from build123d import *

# Parameters (mm, degrees)
F1_DEPTH = 25.4
F4_DEPTH = 15.875


with BuildPart() as f1:
    # F0 (on Front) → F1 (new body)
    with BuildSketch(Plane.XZ):
        with BuildLine():
            Line((1860.5442472816, 17.4135072052), (-120.6557527184, 17.4135072052))
            Line((-120.6557527184, 17.4135072052), (-120.6557527184, -58.7864927948))
            ThreePointArc((-120.6557527184, -58.7864927948), (869.9442472816, -7.9864927948), (1860.5442472816, -58.7864927948))
            Line((1860.5442472816, -58.7864927948), (1860.5442472816, 17.4135072052))
        make_face()
    extrude(amount=F1_DEPTH)


with BuildPart() as f4:
    # F3 (on Front) → F4 (new body)
    with BuildSketch(Plane.XZ):
        with BuildLine():
            Line((1910.8698048711, -377.0609709263), (-70.3301951289, -377.0609709263))
            Line((-70.3301951289, -377.0609709263), (-70.3301951289, -478.6609709263))
            ThreePointArc((-70.3301951289, -478.6609709262), (920.2698048711, -427.8609709262), (1910.8698048711, -478.6609709262))
            Line((1910.8698048711, -478.6609709263), (1910.8698048711, -377.0609709263))
        make_face()
    extrude(amount=F4_DEPTH)


solid = f4.part
Source: CAD feature listing. Evaluate the final solid. Frame: model axes, mm. Coordinates: 2 decimals unless noted, no trailing zeros. Write each loop counter-clockwise with the first axis right and the second up, starting at its lowest first coordinate (ties: lowest second). Pieces come first, ordered by that corner, then holes. Notation, with made-up numbers: M -25.75,87.5 L -19.75,87.5 A19 ccw -19.75,91.5 Z; hole C 62,-10 d8. An arc over 180 degrees is marked long. Use a Markdown table: item, result.
1) Ray query, L1, parallel to Z at x = 938, y = -7.25; L2, parallel to Z at x = 48, y = -2.25. Return the intervals inside material, ascending.
Conclusion:
| item | result |
|---|---|
| L1 | z = -427.88 to -377.06 |
| L2 | z = -467.23 to -377.06 |
2) Mould query, pull axis X, two halves, no side actions, for faces 1 (the flat face through (906, -15.875, -416)), 2 (the cylindrical face through (906.38, -7.83, -427.87)). Classes: pulls with the +X half, pulls with the -X half, needs draft (parallel to the pull), parting line crosses it, or undercut.
Conclusion:
| item | result |
|---|---|
| face 1 | needs draft |
| face 2 | undercut |
3) Section C-C, the plane x = 1274. Output: boundary loops of the cut face in (y, z) (3 decimals), then the cut area to 3 significant figures.
Conclusion:
| item | result |
|---|---|
| outline | M -15.875,-434.324 L 0,-434.324 L 0,-377.061 L -15.875,-377.061 Z |
| area | 909 mm^2 |
4) Section B-B, the plane y = -11. Output: boundary loops of the cut face in (x, z).
Conclusion:
| item | result |
|---|---|
| outline | M -70.33,-478.66 A9683.75 cw 1910.87,-478.66 L 1910.87,-377.06 L -70.33,-377.06 Z |
